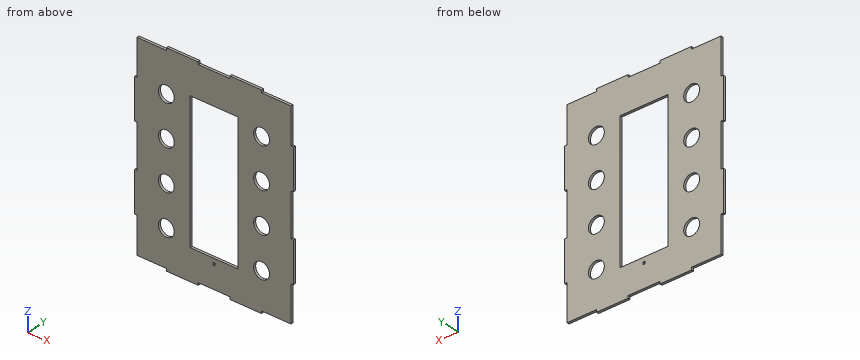
from build123d import *

# Parameters (mm, degrees)
BOSS_EXTRUDE1_DEPTH = 3
SKETCH2_R           = 10
SKETCH2_W           = 60
SKETCH2_H           = 170
CUT_EXTRUDE1_DEPTH  = 162.672508486


with BuildPart() as part:
    # Sketch1 → Boss-Extrude1 (new body)
    with BuildSketch(Plane(origin=(0, 0, 0), x_dir=(1, 0, 0), z_dir=(0, 1, 0))):
        Polygon((20, 123.132735738), (60, 123.132735738), (60, 120.132735738), (97, 120.132735738), (97, 75.132735738), (100, 75.132735738), (100, 25.132735738), (97, 25.132735738), (97, -28.867264262), (100, -28.867264262), (100, -78.867264262), (97, -78.867264262), (97, -123.867264262), (60.028527915, -123.867264262), (60.028527915, -127), (20.028527915, -127), (20.028527915, -124), (-19.971472085, -123.867399906), (-20, -126.867264262), (-60, -126.867264262), (-60.028027258, -123.867395186), (-97, -123.867264262), (-97, -78.867264262), (-100, -78.867264262), (-100, -28.867264262), (-97, -28.867264262), (-97, 25.132735738), (-100, 25.132735738), (-100, 75.132735738), (-97, 75.132735738), (-97, 120.132735738), (-60, 120.132735738), (-60, 123.132735738), (-20, 123.132735738), (-20, 120.132735738), (20, 120.132735738), align=None)
    extrude(amount=BOSS_EXTRUDE1_DEPTH)

    # Sketch2 → Cut-Extrude1 (cut, through all)
    with BuildSketch(Plane(origin=(0, 3, 0), x_dir=(1, 0, 0), z_dir=(0, 1, 0))):
        with Locations(Location((-60.028027258, 75.132735738, 0), (0, 0, 270))):
            Circle(SKETCH2_R)
        with Locations(Location((59.971972742, 75.132735738, 0), (0, 0, 270))):
            Circle(SKETCH2_R)
        with Locations(Location((-60.028027258, 25.132735738, 0), (0, 0, 270))):
            Circle(SKETCH2_R)
        with Locations(Location((59.971972742, 25.132735738, 0), (0, 0, 270))):
            Circle(SKETCH2_R)
        with Locations(Location((-60.028027258, -24.867264262, 0), (0, 0, 270))):
            Circle(SKETCH2_R)
        with Locations(Location((59.971972742, -24.867264262, 0), (0, 0, 270))):
            Circle(SKETCH2_R)
        with Locations(Location((-60.028027258, -74.867264262, 0), (0, 0, 270))):
            Circle(SKETCH2_R)
        with Locations(Location((59.971972742, -74.867264262, 0), (0, 0, 270))):
            Circle(SKETCH2_R)
        Rectangle(SKETCH2_W, SKETCH2_H)
        Polygon((0, 90), (-1.5, 90), (-1.5, 93), (1.5, 93), (1.5, 90), align=None)
    extrude(amount=-CUT_EXTRUDE1_DEPTH, mode=Mode.SUBTRACT)


solid = part.part
Source: CAD feature listing. Evaluate the final solid. Frame: model axes, mm. Coordinates: 2 decimals unless noted, no trailing zeros. Order: outer loops, then holes, each group sorted by start corner. A loop starts at its lowest first (then second) coordinate and runs counter-clockwise, first axis right, second up. Notation, with made-up numbers: M 60,10.5 L 83,10.5 A10 cw 83,14.5 Z; hole C 30.25,-23 d3. An arc over 180 degrees is marked long. Write each question's results on one line, items separated by ' | '. Start each with the question number.
1. Section B-B, the plane x = -24.5. Return the cut outline in (y, z), then the cut area to 3 significant figures.
2. Section D-D, the plane x = 55. Return the cut outline in (y, z).
3. Material intervals for L1, parallel to X at y = 0.35, z = -25; L2, parallel to Z at x = 29, y = 1.9; L3, parallel to X at y = 2.35, z = -39.5, sorted ascending.
4. Section C-C, the plane z = -22. Return the cut outline in (x, y).
5. Pin query (flat end, axial travel): pin 1 (1.5 mm diameter, centred on x = 99, y = 1.5, fed in from -Z); pin 2 (1.5 mm diameter, centred on x = 98, y = 1, fed in from +Z); pin 3 (1.5 mm diameter, centred on y = 2.5, z = -83.5, fed in from +X). Return the tip coordinate at first contact, or that it passes through.
6. Section A-A, the plane z = 59.5. Return the cut outline in (x, y).
Solution:
1) outline: M 0,-123.13 L 3,-123.13 L 3,-85 L 0,-85 Z; M 0,85 L 3,85 L 3,126.87 L 0,126.87 Z | area: 240 mm²
2) outline: M 0,-123.13 L 3,-123.13 L 3,-83.81 L 0,-83.81 Z; M 0,-66.46 L 3,-66.46 L 3,-33.81 L 0,-33.81 Z; M 0,-16.46 L 3,-16.46 L 3,16.19 L 0,16.19 Z; M 0,33.54 L 3,33.54 L 3,66.19 L 0,66.19 Z; M 0,83.54 L 3,83.54 L 3,127 L 0,127 Z
3) L1: -97 to -70.03, -50.03 to -30, 30 to 49.97, 69.97 to 97 | L2: -123.13 to -85, 85 to 127 | L3: -100 to -30, 30 to 100
4) outline: M -97,0 L -69.52,0 L -69.52,3 L -97,3 Z; M -50.53,0 L -30,0 L -30,3 L -50.53,3 Z; M 30,0 L 50.48,0 L 50.48,3 L 30,3 Z; M 69.47,0 L 97,0 L 97,3 L 69.47,3 Z
5) pin 1: z = -75.13 | pin 2: z = 78.87 | pin 3: x = 97
6) outline: M -100,0 L -30,0 L -30,3 L -100,3 Z; M 30,0 L 100,0 L 100,3 L 30,3 Z
